Autodesk Inventor part; units mm, degrees
ref_plane "body_screw_XY" through (5, -10, 0) normal (1, 0, 0) x (0, 0, -1)
ref_plane "body_screw_YZ" through (5, -10, 0) normal (0, 0, -1) x (0, 1, 0)
ref_plane "body_screw_ZX" through (5, -10, 0) normal (0, 1, 0) x (1, 0, 0)
sketch "Sketch_1" plane through (0, 0, 0) normal (1, 0, 0) x (0, 1, 0)
  line L0 (0, -5) -> (0, 6.5)
  line L1 (7.5, 6.5) -> (6.5, 6.5)
  line L2 (6.5, 6.5) -> (6, 6)
  line L3 (6, 6) -> (6, -4.5)
  line L4 (6, -4.5) -> (6.5, -5)
  line L5 (6.5, -5) -> (14.5, -5)
  line L6 (14.5, -5) -> (15, -4.5)
  line L7 (15, -4.5) -> (15, 4.5)
  line L8 (15, 4.5) -> (14.5, 5)
  line L9 (14.5, 5) -> (8, 5)
  line L10 (8, 5) -> (8, 6)
  line L11 (8, 6) -> (7.5, 6.5)
revolve "Revolution1" add sketch "Sketch_1" angle 360 about axis through (0, 0, -5) along (0, 0, -1)
sketch "Sketch_2" plane through (0, 0, 0) normal (0, 0, 1) x (1, 0, 0)
  line L0 (-0.75, -15) -> (0.75, -15)
  line L1 (0.75, -15) -> (0.75, 0)
  line L2 (0.75, 0) -> (-0.75, 0)
  line L3 (-0.75, 0) -> (-0.75, -15)
extrude "Extrusion1" cut sketch "Sketch_2" along normal mid plane 23
sketch "Sketch_3" plane through (0, 0, 0) normal (0, 0, 1) x (1, 0, 0)
  line L0 (0, -10) -> (15, -10)
  line L1 (15, -10) -> (15, -13.75)
  line L2 (15, -13.75) -> (5, -13.75)
  line L3 (5, -13.75) -> (5, -12.25)
  line L4 (5, -12.25) -> (0, -12.25)
  line L5 (0, -12.25) -> (0, -10)
  line L6 (0, -10) -> (15, -10)
revolve "Revolution2" cut sketch "Sketch_3" angle 360 about axis through (0, -10, 0) along (1, 0, 0)
sketch "Sketch4" plane through (-0.75, -14.4806, -5) normal (1, 0, 0) x (0, 0, -1)
  point P0 (-5, 4.4806)
hole "Hole1" at (-0.75, -10, 0) direction (-1, 0, 0) diameter 3.242 depth 15
sketch "_____1" plane through (0, 0, 0) normal (0, 0, 1) x (1, 0, 0)
  line L0 (10.6235, 6.9995) -> (11.3735, 5.7005)
  line L1 (11.3735, 5.7005) -> (13.3654, 6.8505)
  line L2 (13.3654, 6.8505) -> (12.6154, 8.1495)
  line L3 (12.6154, 8.1495) -> (10.6235, 6.9995)
extrude "Extrusion2" cut sketch "_____1" along normal mid plane 10
ref_plane "body_screw_XY" through (5, -10, 0) normal (1, 0, 0) x (0, 0, -1)
ref_plane "body_screw_YZ" through (5, -10, 0) normal (0, 0, -1) x (0, 1, 0)
ref_plane "body_screw_ZX" through (5, -10, 0) normal (0, 1, 0) x (1, 0, 0)
properties part number "C-SCSBNAW12-16_b"
Can you work these out from the model? Positions are in its coordinate system, mm. A direction names the side the tool comes from. Round coordinates to 2 decimals unless told otherwise and drop trailing zeros. Order: outer loops, then holes, each group sorted by start corner. A loop starts at its lowest first (then second) coordinate and runs counter-clockwise, first axis right, second up.
(1) We'd pull the mould along Z, two halves only. Please class faces 4 (the face through (12.347, 6.263, -0.07)), 5 (the face through (2.845, -7.752, 0.099)), 6 (the face through (-3, 6, -5)): +Z half, -Z half, draft (parallel to the pull), parting line (faces both ways), or undercut.
Results are:
face 4: draft
face 5: undercut
face 6: -Z half
(2) If we section it at A-A (z = 0): Please give me the cut outline in (x, y).
Results are:
outline: (-12.44, -8.38) - (-0.75, -8.38) - (-0.75, -5.95) arc R6 cw (long way) to (0.75, -5.95) - (0.75, -7.75) - (5, -7.75) - (5, -6.25) - (13.64, -6.25) arc R15 ccw to (13.35, 6.84) - (11.37, 5.7) - (10.62, 7) - (12.6, 8.14) arc R15 ccw (long way) to start; (-9.48, -11.62) arc R15 ccw to (-0.75, -14.98) - (-0.75, -11.62) - close; (0.75, -14.98) arc R15 ccw to (5.99, -13.75) - (5, -13.75) - (5, -12.25) - (0.75, -12.25) - close
(3) On a 3-axis mill with a long thin cutter (end or side, diameter ignored), from which of +Z, -Z, +X, -X, +Y, -Y can I reach the whole of each face in a straight line? I mean faces 1 (the face through (11.63, 7.58, -0.07)), 2 (the face through (0.341, 7.993, 5.507)), 3 (the face through (0.75, -12, 2)). Say none if no direction works.
Results are:
face 1: +Z, -Z, +X
face 2: +Z
face 3: +Z, -Z, -Y
(4) If we section it at B-B (x = 2.5): Count the separate pieces of the cut face and the enclosed holes in it, plus the area to 3 significant figures.
Results are:
separate pieces: 2
enclosed holes: 1
area: 176 mm2
(5) If I drill on L1, parallel to Z at x = 4.05, y = -10; L2, parallel to Y at x = -3.5, z = 0; L3, parallel to Y at x = 2.6, z = 0, over which ranges is the centre line in solid material (lowest first)?
Results are:
L1: z = -5 to -2.25, 2.25 to 5
L2: y = -14.59 to -11.62, -8.38 to -4.87, 4.87 to 14.59
L3: y = -14.77 to -12.25, -7.75 to -5.41, 5.41 to 14.77
(6) I'm going to push flat-ended pins straight in: pin 1 (4 mm diameter, centred on y = -10, z = 0, fed in from -X); pin 2 (2 mm diameter, centred on x = -7.5, z = 1, fed in from -Y); pin 3 (3 mm diameter, centred on x = -4.5, z = 1, fed in from +Y). Where does each tip first touch, or does it pass through?
Results are:
pin 1: stops at x = -12.69
pin 2: stops at y = -13.52
pin 3: stops at y = 14.7
